Answer from the drawing. Dimensions are ordinates in mm from the lowest x, y and z of the part. Coordinates: 2 decimals unless noted, no trailing zeros. Order: outer loops, then holes, each group sorted by start corner. A loop starts at its lowest first (then second) coordinate and runs counter-clockwise, first axis right, second up. Notation, with made-up numbers: M 85.5,-12.5 L 134.5,-12.5 A13 ccw 134.5,-4.5 Z; hole C -5.75,-20 d4. An arc over 180 degrees is marked long. Use a Markdown table: item, result.
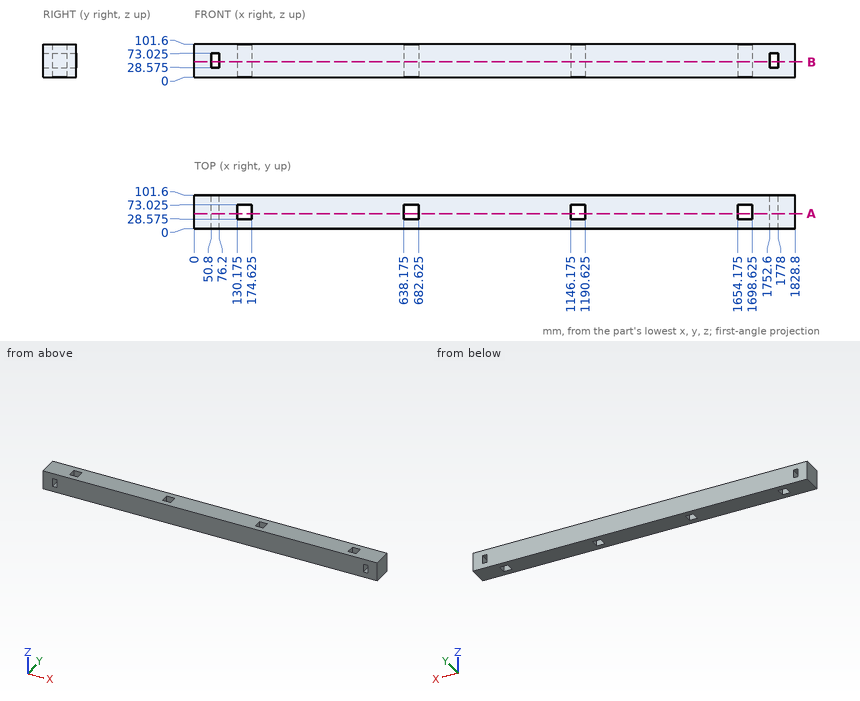
(1) Straight lines are drawn through the part: L1, parallel to X at y = 63.5, z = 15.5 (3 decimals); L2, parallel to X at y = 97, z = 34.5; L3, parallel to Y at x = 138.5, z = 57.5 (3 decimals). For each, find the intervals that lie inside material, in ascending order.
Conclusion:
| item | result |
|---|---|
| L1 | 0 to 130.175, 174.625 to 638.175, 682.625 to 1146.175, 1190.625 to 1654.175, 1698.625 to 1828.8 |
| L2 | 0 to 50.8, 76.2 to 1752.6, 1778 to 1828.8 |
| L3 | 0 to 28.575, 73.025 to 101.6 |
(2) A cutting plane is placed at A-A (y = 46). Determine the outline of the cut face in (x, z) (3 decimals), then the cut area to 3 significant figures.
Conclusion:
| item | result |
|---|---|
| outline | M 0,0 L 130.175,0 L 130.175,101.6 L 0,101.6 Z; M 174.625,0 L 638.175,0 L 638.175,101.6 L 174.625,101.6 Z; M 682.625,0 L 1146.175,0 L 1146.175,101.6 L 682.625,101.6 Z; M 1190.625,0 L 1654.175,0 L 1654.175,101.6 L 1190.625,101.6 Z; M 1698.625,0 L 1828.8,0 L 1828.8,101.6 L 1698.625,101.6 Z; hole M 50.8,28.575 L 76.2,28.575 L 76.2,73.025 L 50.8,73.025 Z; hole M 1752.6,28.575 L 1778,28.575 L 1778,73.025 L 1752.6,73.025 Z |
| area | 165,000 mm2 |
(3) Given P1, Ø1.5, axis at x = 391, z = 63.5, coming from the -Y side, flat-ended and moving along its own axis, determine where the tip first touches the part or whether it passes through.
Conclusion:
| item | result |
|---|---|
| P1 | y = 0 |
(4) A cutting plane is placed at B-B (z = 47.5). Determine the outline of the cut face in (x, y) (3 decimals), then the cut area to 3 significant figures.
Conclusion:
| item | result |
|---|---|
| outline | M 0,0 L 50.8,0 L 50.8,101.6 L 0,101.6 Z; M 76.2,0 L 1752.6,0 L 1752.6,101.6 L 76.2,101.6 Z; M 1778,0 L 1828.8,0 L 1828.8,101.6 L 1778,101.6 Z; hole M 130.175,28.575 L 174.625,28.575 L 174.625,73.025 L 130.175,73.025 Z; hole M 638.175,28.575 L 682.625,28.575 L 682.625,73.025 L 638.175,73.025 Z; hole M 1146.175,28.575 L 1190.625,28.575 L 1190.625,73.025 L 1146.175,73.025 Z; hole M 1654.175,28.575 L 1698.625,28.575 L 1698.625,73.025 L 1654.175,73.025 Z |
| area | 173,000 mm2 |
